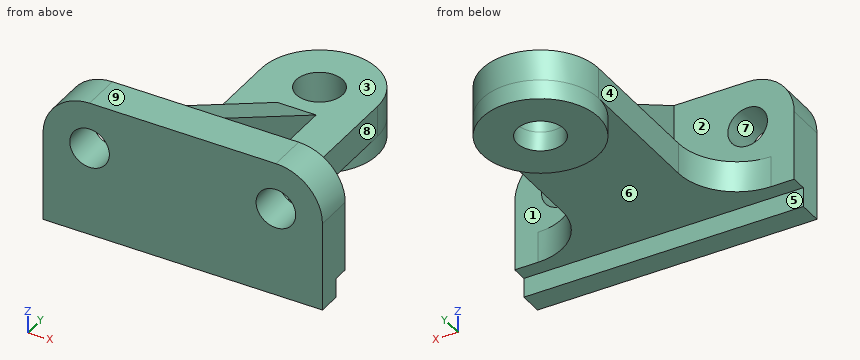
from build123d import *

# Parameters (mm, degrees)
SKETCH1_W           = 72
SKETCH1_H           = 35
BOSS_EXTRUDE1_DEPTH = 10
FILLET1_R           = 12
SKETCH2_W           = 5
SKETCH2_H           = 4
CUT_EXTRUDE1_DEPTH  = 75.767974428
SKETCH3_R           = 6
BOSS_EXTRUDE2_DEPTH = 8
FILLET2_R           = 15
FILLET3_R           = 15
M12_TAPPED_HOLE1_D  = 10.2
SKETCH7_R           = 15
SKETCH7_R_2         = 6
BOSS_EXTRUDE3_DEPTH = 5
RIB1_REACH          = 87.013
SKETCH8_WALL_W      = 217.67731737
SKETCH8_WALL_H      = 10


with BuildPart() as part:
    # Sketch1 → Boss-Extrude1 (new body)
    with BuildSketch(Plane(origin=(0, 0, 0), x_dir=(1, 0, 0), z_dir=(0, 1, 0))):
        Rectangle(SKETCH1_W, SKETCH1_H)
    extrude(amount=BOSS_EXTRUDE1_DEPTH)

    # Fillet1
    fillet1_edges = [part.edges().sort_by_distance(p)[0] for p in [
        (36, 5, 17.5),
        (-36, 5, 17.5),
    ]]
    fillet(fillet1_edges, radius=FILLET1_R)

    # Sketch2 → Cut-Extrude1 (cut, through all)
    with BuildSketch(Plane(origin=(36, 0, 0), x_dir=(0, 0, -1), z_dir=(1, 0, 0))):
        with Locations((15, 8)):
            Rectangle(SKETCH2_W, SKETCH2_H)
    extrude(amount=-CUT_EXTRUDE1_DEPTH, mode=Mode.SUBTRACT)

    # Sketch3 → Boss-Extrude2 (add)
    with BuildSketch(Plane(origin=(0, 0, -12.5), x_dir=(-1, 0, 0), z_dir=(0, 0, -1))):
        with BuildLine():
            Line((15, 10), (-15, 10))
            Line((-15, 10), (-15, 60))
            ThreePointArc((-15, 60), (0, 75), (15, 60))
            Line((15, 60), (15, 10))
        make_face()
        with Locations((0, 60)):
            Circle(SKETCH3_R, mode=Mode.SUBTRACT)
    extrude(amount=-BOSS_EXTRUDE2_DEPTH)

    # Fillet2
    fillet2_edges = [part.edges().sort_by_distance(p)[0] for p in [
        (15, 10, -8.5),
    ]]
    fillet(fillet2_edges, radius=FILLET2_R)

    # Fillet3
    fillet3_edges = [part.edges().sort_by_distance(p)[0] for p in [
        (-15, 10, -8.5),
    ]]
    fillet(fillet3_edges, radius=FILLET3_R)

    # M12 Tapped Hole1 (through all)
    with Locations(Plane(origin=(0, 10, 0), x_dir=(1, 0, 0), z_dir=(0, 1, 0))):
        with Locations((24, -5.5), (-24, -5.5)):
            Hole(M12_TAPPED_HOLE1_D / 2)

    # Sketch7 → Boss-Extrude3 (add)
    with BuildSketch(Plane(origin=(0, 0, -12.5), x_dir=(-1, 0, 0), z_dir=(0, 0, -1))):
        with Locations((0, 60)):
            Circle(SKETCH7_R)
        with Locations((0, 60)):
            Circle(SKETCH7_R_2, mode=Mode.SUBTRACT)
    extrude(amount=BOSS_EXTRUDE3_DEPTH)

    # Sketch8 wall → Rib1 (add, up to next)
    with BuildSketch(Plane(origin=(0, 30, 6.5), x_dir=(0, 0.876215908677, -0.481918749772), z_dir=(0, 0.481918749772, 0.876215908677)), mode=Mode.PRIVATE) as rib1_sk1:
        Rectangle(SKETCH8_WALL_W, SKETCH8_WALL_H)
    rib1_tool1 = extrude(rib1_sk1.sketch, amount=-RIB1_REACH, mode=Mode.PRIVATE) - part.part
    add(rib1_tool1.solids().sort_by_distance((0, 30, 6.5))[0])


solid = part.part
Verification items for the finished model (mm, model axes). Face numbers are marked on the shaded views. A direction names the side the tool comes from. Give positions to 0.01 mm unless a question says otherwise; leave off trailing zeros. Order: outer loops, then holes, each group sorted by start corner. A loop starts at its lowest first (then second) coordinate and runs counter-clockwise, first axis right, second up. Notation, with made-up numbers: M 54.5,76.25 L 101.5,76.25 A8 cw 101.5,90.25 Z; hole C 46,-5 d8. An arc over 180 degrees is marked long. Answer as a JSON object with one key per item and string values. Group by question number.
1) Scan lines: line 1 along Z through (x, y) = (-24, 4); line 2 along Y through (x, z) = (0, -13); line 3 along X through (y, z) = (4, 5). Record each from-to range of solid material in increasing order. Write a range as [from, to].
2) Cross-section at B-B (z = 2). Enter the section's corners in (x, y), then the cut area to 3 significant figures.
3) Cross-section at A-A (x = 0). Enter the section's corners in (y, z).
4) Cross-section at D-D (y = 43). Enter the section's corners in (x, z), then the cut area to 4 significant figures.
5) Access from +Z, -Z, +X, -X, +Y, -Y to the whole of each face (thin tool, end or side, straight path). Record for the marked faces 1, 2, 3, 4 and 5.
6) Mould release check, pull along Z, two halves, no side actions. Record for the marked faces 6, 7, 8 and 9: released by +Z, released by -Z, zero draft, split by the parting line, or undercut.
7) Depth check by flat-ended pin: pin 1 Ø10 at (y, z) = (41.5, 2) entering from +X; pin 2 Ø4 at (y, z) = (67, -12.5) entering from +X; pin 3 Ø13.5 at (x, z) = (24, 5.5) entering from +Y; pin 4 Ø10 at (x, y) = (23, 51.5) entering from +Z. Enter the tip coordinate at first touch or a pass-through.
8) Cross-section at C-C (z = -10.5). Enter the section's corners in (x, y), then the cut area to 3 significant figures.
Result sheet:
{
 "1": {"line 1": "z = [-17.5, 0.4], [10.6, 17.5]", "line 2": "y = [0, 6], [45, 54], [66, 75]", "line 3": "x = [-36, -29.08], [-18.92, 18.92], [29.08, 36]"},
 "2": {"outline": "M -36,0 L -27.71,0 L -27.71,10 L -36,10 Z; M -20.29,0 L 20.29,0 L 20.29,10 L 5,10 L 5,38.18 L -5,38.18 L -5,10 L -20.29,10 Z; M 27.71,0 L 36,0 L 36,10 L 27.71,10 Z", "area": "853 mm2"},
 "3": {"outline": "M 0,-17.5 L 6,-17.5 L 6,-12.5 L 45,-12.5 L 45,-17.5 L 54,-17.5 L 54,-4.5 L 50,-4.5 L 10,17.5 L 0,17.5 Z; M 66,-17.5 L 75,-17.5 L 75,-4.5 L 66,-4.5 Z"},
 "4": {"outline": "M -15,-12.5 L 15,-12.5 L 15,-4.5 L 5,-4.5 L 5,-0.65 L -5,-0.65 L -5,-4.5 L -15,-4.5 Z", "area": "278.5 mm2"},
 "5": {"face 1": "+Z, +X, +Y", "face 2": "+Z, -X, +Y", "face 3": "+Z, +Y", "face 4": "+Z, -Z, -X, +Y", "face 5": "-Z, +X, -X"},
 "6": {"face 6": "released by -Z", "face 7": "undercut", "face 8": "zero draft", "face 9": "released by +Z"},
 "7": {"pin 1": "stops at x = 5", "pin 2": "stops at x = 14.14", "pin 3": "stops at y = 10", "pin 4": "passes through"},
 "8": {"outline": "M -36,0 L 36,0 L 36,10 L 30,10 A15 cw 15,25 L 15,60 A15 ccw -15,60 L -15,25 A15 cw -30,10 L -36,10 Z; hole C 0,60 d12", "area": "2,560 mm2"}
}
